from build123d import *

# Parameters (mm, degrees)
SKETCH1_R           = 25
BOSS_EXTRUDE1_DEPTH = 8.25
SKETCH2_W           = 50
SKETCH2_H           = 50
BOSS_EXTRUDE2_DEPTH = 5
SKETCH3_R           = 4.5
SKETCH3_R_2         = 1.75
CUT_EXTRUDE1_DEPTH  = 37.305130491
SKETCH5_R           = 3.5
CUT_EXTRUDE3_DEPTH  = 4
CIRPATTERN2_COUNT   = 4
CHAMFER2_SIZE       = 0.5
SKETCH6_W           = 50
SKETCH6_H           = 5
BOSS_EXTRUDE3_DEPTH = 5
SKETCH7_R           = 2.6
CUT_EXTRUDE4_DEPTH  = 40.37003937
CHAMFER3_SIZE       = 1


with BuildPart() as part:
    # Sketch1 → Boss-Extrude1 (new body)
    with BuildSketch(Plane.XY):
        Circle(SKETCH1_R)
    extrude(amount=BOSS_EXTRUDE1_DEPTH)

    # Sketch2 → Boss-Extrude2 (add)
    with BuildSketch(Plane.XY.offset(8.25)):
        Rectangle(SKETCH2_W, SKETCH2_H)
    extrude(amount=-BOSS_EXTRUDE2_DEPTH)

    # Sketch3 → Cut-Extrude1 (cut, through all)
    with BuildSketch(Plane(origin=(0, 0, 0), x_dir=(-1, 0, 0), z_dir=(0, 0, -1))):
        with Locations((12.5, 0)):
            Circle(SKETCH3_R)
        with Locations((-12.5, 0)):
            Circle(SKETCH3_R)
        with Locations((-14.142135624, 14.142135624)):
            Circle(SKETCH3_R_2)
        with Locations((14.142135624, 14.142135624)):
            Circle(SKETCH3_R_2)
        with Locations((14.142135624, -14.142135624)):
            Circle(SKETCH3_R_2)
        with Locations((-14.142135624, -14.142135624)):
            Circle(SKETCH3_R_2)
    extrude(amount=-CUT_EXTRUDE1_DEPTH, mode=Mode.SUBTRACT)

    # Sketch5 → Cut-Extrude3 (cut)
    with BuildSketch(Plane.XY.offset(8.25)):
        with Locations((-14.142135624, 14.142135624)):
            Circle(SKETCH5_R)
    cut_extrude3 = extrude(amount=-CUT_EXTRUDE3_DEPTH, mode=Mode.SUBTRACT)

    # CirPattern2: Cut-Extrude3 ×4 about axis
    cirpattern2_axis = Axis((0, 0, 0), (0, 0, 1))
    for i in range(1, CIRPATTERN2_COUNT):
        add(cut_extrude3.rotate(cirpattern2_axis, i * 360 / CIRPATTERN2_COUNT), mode=Mode.SUBTRACT)

    # Chamfer2
    chamfer2_edges = [part.edges().sort_by_distance(p)[0] for p in [
        (-25, 0, 0),
        (17, 0, 0),
        (15.892135624, 14.142135624, 0),
        (-12.392135624, 14.142135624, 0),
        (-12.392135624, -14.142135624, 0),
        (15.892135624, -14.142135624, 0),
        (-8, 0, 0),
    ]]
    chamfer(chamfer2_edges, length=CHAMFER2_SIZE)

    # Sketch6 → Boss-Extrude3 (add)
    with BuildSketch(Plane.XY.offset(8.25)):
        with Locations((0, 27.5)):
            Rectangle(SKETCH6_W, SKETCH6_H)
        with Locations((0, -27.5)):
            Rectangle(SKETCH6_W, SKETCH6_H)
    extrude(amount=-BOSS_EXTRUDE3_DEPTH)

    # Sketch7 → Cut-Extrude4 (cut, through all)
    with BuildSketch(Plane(origin=(0, 0, 3.25), x_dir=(-1, 0, 0), z_dir=(0, 0, -1))):
        with Locations((-20, 25.5)):
            Circle(SKETCH7_R)
        with Locations((20, 25.5)):
            Circle(SKETCH7_R)
        with Locations((20, -25.5)):
            Circle(SKETCH7_R)
        with Locations((-20, -25.5)):
            Circle(SKETCH7_R)
    extrude(amount=-CUT_EXTRUDE4_DEPTH, mode=Mode.SUBTRACT)

    # Chamfer3
    chamfer3_edges = [part.edges().sort_by_distance(p)[0] for p in [
        (-25, 30, 5.75),
        (25, 30, 5.75),
        (-25, -30, 5.75),
        (25, -30, 5.75),
        (22.6, -25.5, 8.25),
        (22.6, -25.5, 3.25),
        (-17.4, -25.5, 8.25),
        (-17.4, -25.5, 3.25),
        (-17.4, 25.5, 8.25),
        (-17.4, 25.5, 3.25),
        (22.6, 25.5, 8.25),
        (22.6, 25.5, 3.25),
    ]]
    chamfer(chamfer3_edges, length=CHAMFER3_SIZE)


solid = part.part
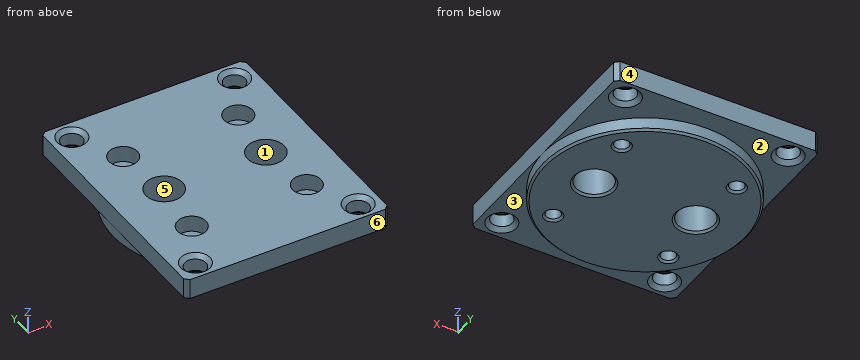
The listing builds one solid part. Answer for the finished solid, in the listing's coordinates (mm). Face numbers are marked on the shaded views. A direction names the side the tool comes from. Give positions to 0.01 mm unless a question says otherwise; leave off trailing zeros. Write each loop counter-clockwise with the first axis right and the second up, starting at its lowest first coordinate (ties: lowest second). Pieces come first, ordered by that corner, then holes.
1) Section B-B (x = 0) is taken. Write down the section's boundary in (y, z).
2) For a pull along Y with two mould halves and no side action, classify the marked faces 4, 5 and 6 as pulls with the +Y half, pulls with the -Y half, needs draft (parallel to the pull), parting line crosses it, or undercut.
3) Section C-C (y = -3) is taken. Count the separate pieces of the cut face and the enclosed holes in it, and give its area (3 significant figures).
4) A tool of negligible diameter and unlimited length cuts with its end or side. For the marked faces 1, 2 and 3, from which of +Z, -Z, +X, -X, +Y, -Y can it reach the whole face along a straight path? Write none if from no direction.
5) Section A-A (z = 2.5) is taken. Write down the section's boundary in (x, y), and give its area (3 significant figures).
6) Find the intervals of material crossed by L1, parallel to Y at x = 22, z = 5.5; L2, parallel to X at y = -14.5, z = 2; L3, parallel to Y at x = -13, z = 3, in increasing order.
7) Given P1, Ø15, axis at x = 1.5, y = -11.5, coming from the -Z side; P2, Ø6, axis at x = -20, y = 25.5, coming from the +Z side; P3, Ø4, axis at x = 7.5, z = 1, coming from the -Y side; P4, Ø7, axis at x = 20, y = -25.5, coming from the +Z side, each flat-ended and moving along its own axis, determine where each tip first touches the part or whether it passes through.
Response:
1. outline: (-30, 3.25) - (-25, 3.25) - (-25, 0.5) - (-24.5, 0) - (24.5, 0) - (25, 0.5) - (25, 3.25) - (30, 3.25) - (30, 8.25) - (-30, 8.25) - close
2. face 4: pulls with the +Y half
2. face 5: undercut
2. face 6: pulls with the -Y half
3. separate pieces: 3
3. enclosed holes: 0
3. area: 300 mm2
4. face 1: +Z, -Z
4. face 2: -Z, +Y
4. face 3: -Z, -Y
5. outline: circle Ø50 at (0, 0); hole circle Ø9 at (-12.5, 0); hole circle Ø3.5 at (-14.14, -14.14); hole circle Ø3.5 at (-14.14, 14.14); hole circle Ø9 at (12.5, 0); hole circle Ø3.5 at (14.14, -14.14); hole circle Ø3.5 at (14.14, 14.14)
5. area: 1,800 mm2
6. L1: y = -30 to -27.16, -23.84 to 23.84, 27.16 to 30
6. L2: x = -20.37 to -15.86, -12.43 to 12.43, 15.86 to 20.37
6. L3: y = -21.35 to -15.47, -12.82 to -4.47, 4.47 to 12.82, 15.47 to 21.35
7. P1: stops at z = 0
7. P2: stops at z = 7.65
7. P3: stops at y = -24.39
7. P4: stops at z = 8.15
